Could you check a few things on this model? Use its own coordinates, in mm. Face numbers are marked on the shaded views. A direction names the side the tool comes from. Give positions to 0.01 mm unless a question says otherwise; leave off trailing zeros. Write each loop counter-clockwise with the first axis right and the second up, starting at its lowest first coordinate (ties: lowest second). Pieces come first, ordered by that corner, then holes. Notation, with made-up numbers: M 74.5,16.5 L 116.5,16.5 A21 cw 116.5,23.5 Z; hole C -23,47.25 d11. An arc over 180 degrees is marked long. One line per item, written item: value.
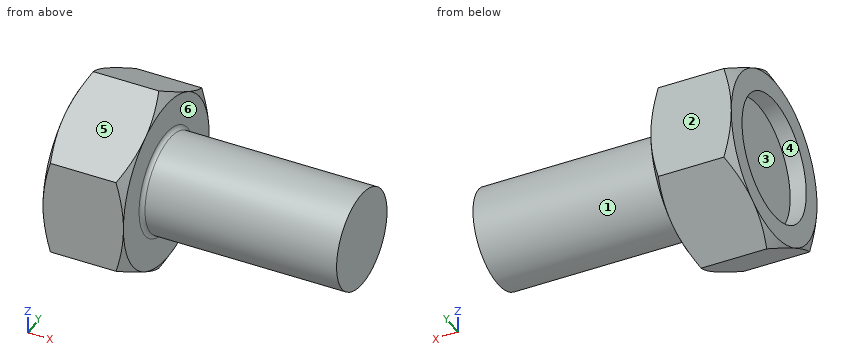
Autodesk Inventor part; units mm, degrees
ref_plane "Work Plane1" through (3, 0, 0) normal (0, 0.5, 0.8660254) x (1, 0, 0)
ref_plane "YZ Plane" through (0, 0, 0) normal (1, 0, 0) x (0, 1, 0)
ref_plane "XZ Plane" through (0, 0, 0) normal (0, 1, 0) x (-1, 0, 0)
sketch "Sketch1" plane through (0, 0, 0) normal (0, 0, 1) x (1, 0, 0)
  line L0 (0, 5) -> (0, 0)
  line L1 (0, 0) -> (20, 0)
  line L2 (20, 0) -> (20, 5)
  line L3 (20, 5) -> (0, 5)
  line L4 (-4, 0) -> (24, 0)
  line L5 (0, -1) -> (0, 6)
  dimension "d0" = 10
  dimension "d1" = 20
revolve "Body" add sketch "Sketch1" angle 360 about axis through (0, 0, 0) along (1, 0, 0)
sketch "Sketch2" plane through (0, 0, 0) normal (1, 0, 0) x (0, 1, 0)
  line L0 (0, 9.815) -> (8.5, 4.9075)
  line L1 (8.5, 4.9075) -> (8.5, -4.9075)
  line L2 (8.5, -4.9075) -> (0, -9.815)
  line L3 (0, -9.815) -> (-8.5, -4.9075)
  line L4 (-8.5, -4.9075) -> (-8.5, 4.9075)
  line L5 (-8.5, 4.9075) -> (0, 9.815)
  line L6 (-11.9, 0) -> (11.9, 0)
  line L7 (0, -13.7409) -> (0, 13.7409)
  point P0 (0, 0)
  point P1 (0, 0)
  dimension "d2" = 17
extrude "Head" add sketch "Sketch2" against normal blind 8.23
sketch "Sketch3" plane through (-8.23, 0, 0) normal (-1, 0, 0) x (0, 1, 0)
  circle A0 centre (0, 0) radius 6.375
  point P0 (0, 0)
  dimension "d12" = 12.75
extrude "Indent1" cut sketch "Sketch3" against normal blind 1.646
sketch "Sketch4" plane through (0, 0, 0) normal (0, 0, 1) x (1, 0, 0)
  line L0 (-8.23, 9.815) -> (-8.23, 8.5)
  line L1 (-8.23, 8.5) -> (-7.4708, 9.815)
  line L2 (-7.4708, 9.815) -> (-8.23, 9.815)
  line L3 (0, 9.815) -> (0, 8.5)
  line L4 (0, 8.5) -> (-0.7592, 9.815)
  line L5 (-0.7592, 9.815) -> (0, 9.815)
  line L6 (0, 0) -> (-8.23, 0)
  line L7 (-8.23, 0) -> (-8.23, 8.5)
  line L8 (0, 0) -> (0, 8.5)
  line L9 (-9.876, 0) -> (1.646, 0)
  line L10 (-7.4708, 9.815) -> (-0.7592, 9.815) construction
  line L11 (0, -1.963) -> (0, 11.7779)
  dimension "d6" = 30
  dimension "d7" = 30
  dimension "d16" = 17
  dimension "d17" = 17
  dimension "d18" = 19.6299
revolve "Chamfer1" cut sketch "Sketch4" angle 360 about axis through (-10, 0, 0) along (1, 0, 0)
fillet "Fillet1" radius 0.4 1 edges at (0, -5, 0)
thread "Thread"
ref_plane "Work Plane1" through (3, 0, 0) normal (0, 0.5, 0.8660254) x (1, 0, 0)
equation "\"d2\" = SW"
equation "\"d3\" = KOH"
equation "\"d12\" = 0.75 * SW0"
equation "\"d14\" = 0.2 * KOH"
equation "\"d11\" = RR"
equation "\"d8\" = GEL"
equation "\"d0\" = GD"
equation "\"d1\" = NLG"
equation "\"d6\" = ANG1"
equation "\"d7\" = ANG1"
equation "\"d16\" = SW0"
equation "\"d17\" = SW0"
equation "\"d18\" = 1.1547 * SW"
equation "\"NLG\" = 20"
equation "\"KOH\" = 8.23"
equation "\"GD\" = NND"
equation "\"GEL\" = 17"
equation "\"SW\" = 17"
equation "\"SW0\" = SW"
equation "\"ANG1\" = 30deg"
equation "\"RR\" = 0.4"
equation "\"GUL\" = 0.61345 * PTC"
equation "\"SPD\" = NND - 1.2269 * PTC"
equation "\"GD1\" = THREADDIA - 1.2269 * PTC"
equation "\"SDH\" = 11.2"
equation "\"TOA\" = 30deg"
equation "\"FAWI\" = 45deg"
equation "\"PTC\" = 1.5"
equation "\"GAL\" = 0.61345 * PTC"
equation "\"SD\" = 0"
equation "\"SD2\" = SDH"
equation "\"E0\" = 1.155 * SW"
properties part number "AS 1427 - M10 x 20" material "Steel, Mild"
1) We'd pull the mould along Y, two halves only. Please class the marked faces 1, 2, 3 and 4: pulls with the +Y half, pulls with the -Y half, needs draft (parallel to the pull), parting line crosses it, or undercut.
Outcome:
face 1: parting line crosses it
face 2: pulls with the +Y half
face 3: undercut
face 4: undercut
2) Please list where these lines run through material, in increasing order: L1, parallel to Y at x = -7.65, z = 0 (3 decimals); L2, parallel to X at y = -2, z = 0.75; L3, parallel to Z at x = -7.5, y = 0 (3 decimals). Write a range as from..to.
Outcome:
L1: y = -8.5..-6.375, 6.375..8.5
L2: x = -6.58..20
L3: z = -9.764..-6.375, 6.375..9.764
3) I'm going to push flat-ended pins straight in: pin 1 (4 mm diameter, centred on y = -0.5, z = 2.5, fed in from -X); pin 2 (3 mm diameter, centred on x = 6.5, z = -1.5, fed in from +Y); pin 3 (10 mm diameter, centred on x = -0.5, z = -7.5, fed in from +Y); pin 4 (4 mm diameter, centred on x = -1, z = 7, fed in from -Y). Where does each tip first touch, or does it pass through?
Outcome:
pin 1: stops at x = -6.58
pin 2: stops at y = 5
pin 3: stops at y = 8.5
pin 4: stops at y = -8.34
4) If we section it at A-A, the plane x = 12.5: Write out the boundary of the cut face in (y, z).
Outcome:
outline: C 0,0 d10
5) On a 3-axis mill with a long thin cutter (end or side, diameter ignored), from which of +Z, -Z, +X, -X, +Y, -Y can I reach the whole of each face in a straight line? I mean the marked faces 5 and 6. Say none if no direction works.
Outcome:
face 5: +Z, +X, -X, -Y
face 6: +X
